Autodesk Fusion 360 part; units mm, degrees
sketch "Sketch1" plane through (0, 0, 0) normal (0, 0, 1) x (1, 0, 0)
  circle A0 centre (0, 0) radius 7
  circle A1 centre (0, 0) radius 6.15
  circle A2 centre (0, 0) radius 2.05
  line L0 (-1.5, 0) -> (-1.5, -1.3973)
  line L1 (-1.5, 0) -> (-1.5, 1.3973)
  point P0 (-1.5, 0)
  dimension "d1" = 14
  dimension "d2" = 12.3
  dimension "d3" = 4.1
  dimension "d4" = 1.5
extrude "Extrude1" add sketch "Sketch1" along normal blind 1.5 contours A0 | A1 | A2 L0 L1 | A2 L0 L1
extrude "Extrude2" add sketch "Sketch1" along normal blind 25.5 contours A1 | A2 L0 L1 picked at (0.859, -0.1018)
extrude "Extrude3" add sketch "Sketch1" along normal blind 7.5 contours A2 L0 L1 picked at (0.859, -0.1018)
Could you check a few things on this model? Use its own coordinates, in mm. A direction names the side the tool comes from. Give positions to 0.01 mm unless a question says otherwise; leave off trailing zeros. Order: outer loops, then holes, each group sorted by start corner. A loop starts at its lowest first (then second) coordinate and runs counter-clockwise, first axis right, second up. Notation, with made-up numbers: (59.5, 45) - (117.5, 45) arc R14 ccw to (117.5, 72) - close; hole circle Ø1 at (31.25, -11.5). An arc over 180 degrees is marked (long way). Return JSON: item names as keys, results as strings. Group by question number.
Q1. Please list where these lines run through material, in increasing order: line 1 along X through (y, z) = (0, 6.5); line 2 along Z through (x, y) = (-4.5, -4.5); line 3 along X through (y, z) = (-1.5, 10.25). Write a range as [from, to].
Q2. Suppose I cut it at D-D, the plane y = 4.5. Please give me the cut outline in (x, z).
Q3. Suppose I cut it at B-B, the plane x = 0. Please give me the cut outline in (y, z).
Q4. Which directions (+Z, -Z, +X, -X, +Y, -Y) give clear straight access to the entire face, cutting with the end or side of a thin tool? Please do faces 5 (the face through (4, -5, 1.5)), 6 (the face through (6.466, 2.681, 0.74)).
Q5. Suppose I cut it at C-C, the plane z = 17.5. Please give me the cut outline in (x, y).
Q6. Suppose I cut it at A-A, the plane y = 0. Please give me the cut outline in (x, z), and give its area (3 significant figures).
Q7. Thinking about a two-plate mould opening in X: for faces 1 (the face through (-1.333, 6.004, 13.332)), 2 (the face through (-1.5, 0, 13)), 3 (the face through (0, 0, 25.5)), 4 (the face through (-2.05, -0.02, 13.33)), which applies, pulls with the +X half, pulls with the -X half, needs draft (parallel to the pull), parting line crosses it, or undercut?
Q8. Will these pins go through, and if not, where does the flat tip stop? pin 1 Ø1.4 at (y, z) = (0.5, 18.5) entering from -X; pin 2 Ø1 at (x, z) = (1.5, 2.5) entering from -Y; pin 3 Ø1.5 at (y, z) = (-4.5, 15.5) entering from -X; pin 4 Ø5 at (x, y) = (-3.5, 2.5) entering from -Z.
Resolved:
{
 "1": {"line 1": "x = [-6.15, -2.05], [-1.5, 6.15]", "line 2": "z = [0, 1.5]", "line 3": "x = [-5.96, 5.96]"},
 "2": {"outline": "(-5.36, 0) - (5.36, 0) - (5.36, 1.5) - (4.19, 1.5) - (4.19, 25.5) - (-4.19, 25.5) - (-4.19, 1.5) - (-5.36, 1.5) - close"},
 "3": {"outline": "(-7, 0) - (7, 0) - (7, 1.5) - (6.15, 1.5) - (6.15, 25.5) - (-6.15, 25.5) - (-6.15, 1.5) - (-7, 1.5) - close"},
 "4": {"face 5": "+Z", "face 6": "+Z, -Z"},
 "5": {"outline": "circle Ø12.3 at (0, 0); hole (-1.5, -1.4) - (-1.5, 1.4) arc R2.05 ccw to start"},
 "6": {"outline": "(-7, 0) - (7, 0) - (7, 1.5) - (6.15, 1.5) - (6.15, 25.5) - (-1.5, 25.5) - (-1.5, 1.5) - (-2.05, 1.5) - (-2.05, 25.5) - (-6.15, 25.5) - (-6.15, 1.5) - (-7, 1.5) - close", "area": "303 mm2"},
 "7": {"face 1": "parting line crosses it", "face 2": "undercut", "face 3": "needs draft", "face 4": "undercut"},
 "8": {"pin 1": "stops at x = -6.15", "pin 2": "stops at y = -6.07", "pin 3": "stops at x = -4.87", "pin 4": "stops at z = 0"}
}
